from build123d import *

# Parameters (mm, degrees)
BOSS_EXTRUDE1_DEPTH = 50
SKETCH2_W           = 20
SKETCH2_H           = 15
CUT_EXTRUDE1_DEPTH  = 40
CUT_EXTRUDE2_DEPTH  = 134
CUT_EXTRUDE3_REACH  = 85.762
SKETCH5_R           = 3.3


with BuildPart() as part:
    # Sketch1 → Boss-Extrude1 (new body)
    with BuildSketch(Plane(origin=(0, 0, 0), x_dir=(1, 0, 0), z_dir=(0, 1, 0))):
        Polygon((0, 0), (34, 0), (34, 20), (54, 20), (54, 0), (88, 0), (88, -40), (0, -40), align=None)
    extrude(amount=BOSS_EXTRUDE1_DEPTH)

    # Sketch2 → Cut-Extrude1 (cut)
    with BuildSketch(Plane(origin=(54, 0, 0), x_dir=(0, 0, -1), z_dir=(1, 0, 0))):
        with Locations((10, 7.5)):
            Rectangle(SKETCH2_W, SKETCH2_H)
    extrude(amount=-CUT_EXTRUDE1_DEPTH, mode=Mode.SUBTRACT)

    # Sketch3 → Cut-Extrude2 (cut)
    with BuildSketch(Plane(origin=(88, 0, 0), x_dir=(0, 0, -1), z_dir=(1, 0, 0))):
        with BuildLine():
            Line((-40, 0), (-40, 50))
            Line((-40, 50), (-12.980453639, 50))
            add(Edge.make_bspline(
                [(-40, 0), (-14.830140994, 17.978651643), (-12.980453639, 50)],
                knots=[0, 0, 0, 1, 1, 1], degree=2))
        make_face()
    extrude(amount=-CUT_EXTRUDE2_DEPTH, mode=Mode.SUBTRACT)

    # Sketch5 → Cut-Extrude3 (cut, up to next)
    with BuildSketch(Plane(origin=(54, 0, 0), x_dir=(0, 0, -1), z_dir=(1, 0, 0)), mode=Mode.PRIVATE) as cut_extrude3_sk1:
        with Locations((7.5, 42.5)):
            Circle(SKETCH5_R)
    cut_extrude3_tool1 = extrude(cut_extrude3_sk1.sketch, amount=-CUT_EXTRUDE3_REACH, mode=Mode.PRIVATE) & part.part
    # Sketch5 → Cut-Extrude3 (cut, up to next)
    with BuildSketch(Plane(origin=(54, 0, 0), x_dir=(0, 0, -1), z_dir=(1, 0, 0)), mode=Mode.PRIVATE) as cut_extrude3_sk2:
        with Locations((7.5, 27.5)):
            Circle(SKETCH5_R)
    cut_extrude3_tool2 = extrude(cut_extrude3_sk2.sketch, amount=-CUT_EXTRUDE3_REACH, mode=Mode.PRIVATE) & part.part
    add(cut_extrude3_tool1.solids().sort_by_distance((54, 42.5, -7.5))[0], mode=Mode.SUBTRACT)
    add(cut_extrude3_tool2.solids().sort_by_distance((54, 27.5, -7.5))[0], mode=Mode.SUBTRACT)


solid = part.part
Source: CAD feature listing. Evaluate the final solid. Frame: model axes, mm. A direction names the side the tool comes from. Coordinates: 2 decimals unless noted, no trailing zeros. Loops run counter-clockwise (first coordinate to the right, second up) from the corner with the lowest first, then second, coordinate; pieces in that order, holes last. Notation, with made-up numbers: (80.25, 54) - (138.25, 54) arc R14 ccw to (138.25, 61) - close; hole circle Ø3 at (68.25, 56.5). An arc over 180 degrees is marked (long way). One line per item, written item: value. Start each with the question number.
1. Contact query for flat-ended pins moving along their axis: P1, Ø4, axis at x = 60, y = 10.5, coming from the +Z side; P2, Ø1, axis at x = 73.5, y = 15.5, coming from the -Z side; P3, Ø16, axis at y = 36.5, z = -11.5, coming from the -X side. Output: stop coordinate, or through.
2. Section A-A (z = -7.5). Return the cut outline in (x, y), and give its area (3 significant figures).
3. Ray query, L1, parallel to Y at x = 41.5, z = -7.5; L2, parallel to X at y = 48, z = -5; L3, parallel to Z at x = 43, y = 42. Return the intervals inside material, ascending.
4. Mould query, pull axis Y, two halves, no side actions, for faces 1 (the flat face through (44, 32, -20)), 2 (the flat face through (44, 15, -10)), 3 (the cylindrical face through (44.14, 45.77, -7.07)), 4 (the cylindrical face through (44.14, 25.492, -4.881)). Classes: pulls with the +Y half, pulls with the -Y half, needs draft (parallel to the pull), parting line crosses it, or undercut.
5. Section B-B (x = 44.5). State how many separate pieces and enclosed holes the cut face has, and give its area (3 significant figures).
6. Set-up query: faces 5 (the flat face through (34, 32, -10)), 6 (the flat face through (0, 19, 11)), 7 (the flat face through (54, 32, -10)). Return all of +Z, -Z, +X, -X, +Y, -Y with unobstructed straight access to the full face (end or side cutting, diameter ignored); none if empty.
Verdict:
1. P1: stops at z = 30.14
1. P2: stops at z = 0
1. P3: stops at x = 34
2. outline: (34, 15) - (54, 15) - (54, 24.2) - (34, 24.2) - close; (34, 30.8) - (54, 30.8) - (54, 39.2) - (34, 39.2) - close; (34, 45.8) - (54, 45.8) - (54, 50) - (34, 50) - close
2. area: 436 mm2
3. L1: y = 15 to 24.2, 30.8 to 39.2, 45.8 to 50
3. L2: x = 34 to 54
3. L3: z = -20 to -10.76, -4.24 to 13.84
4. face 1: needs draft
4. face 2: pulls with the -Y half
4. face 3: undercut
4. face 4: undercut
5. separate pieces: 1
5. enclosed holes: 2
5. area: 1,700 mm2
6. face 5: -Z, -X, +Y, -Y
6. face 6: +Z, -Z, -X, +Y, -Y
6. face 7: -Z, +X, +Y, -Y
